The model under review builds one solid part; all positions refer to its coordinate system, in mm. A direction names the side the tool comes from. Coordinates: 2 decimals unless noted, no trailing zeros. Order: outer loops, then holes, each group sorted by start corner. A loop starts at its lowest first (then second) coordinate and runs counter-clockwise, first axis right, second up.
```python
from build123d import *

# Parameters (mm, degrees)
F0_R     = 7.5
F0_R_2   = 1.75
F1_DEPTH = 5.05


# Not quite as in the source:
# - a fillet or chamfer that OpenCascade refuses, or shapes differently, is made with other operations: its cross-section is extruded or revolved along the edge and cut away or added


with BuildPart() as f1:
    # F0 (on Top) → F1 (new body)
    with BuildSketch(Plane.XY):
        Circle(F0_R)
        Circle(F0_R_2, mode=Mode.SUBTRACT)
    extrude(amount=F1_DEPTH)

    # F2 (on Front) → F3 (revolve, cut)
    with BuildSketch(Plane.XZ):
        Polygon((3, 1.5), (3, 0), (7.75, 0), (7.75, 3.5), (5, 3.5), (5, 1.5), align=None)
        with BuildLine():
            Line((0, 5.05), (0, 1.8))
            ThreePointArc((0, 1.8), (3.25, 5.05), (0, 8.3))
            Line((0, 8.3), (0, 5.05))
        make_face()
    revolve(axis=Axis((0, 0, 2.525), (0, 0, 1)), mode=Mode.SUBTRACT)

    # F4: chamfer of 2 on 1 edges, made by hand

    # F4_s1 → F4_t2 (revolve, cut)
    with BuildSketch(Plane.XZ):
        with BuildLine():
            Line((4.8541219597, 5.05), (3.0049326417, 3.8119047619))
            ThreePointArc((3.0049326417, 3.8119047619), (3.1823683685, 4.3904307714), (3.25, 5.05))
            Line((3.25, 5.05), (4.8541219597, 5.05))
        make_face()
    revolve(axis=Axis((0, 0, 5.05), (0, 0, 1)), mode=Mode.SUBTRACT)


solid = f1.part
```
(1) For pin 1 Ø8 at (x, y) = (-1, -1.5) entering from -Z; pin 2 Ø3 at (x, y) = (-5, -0.5) entering from -Z; pin 3 Ø2 at (y, z) = (0.5, 1) entering from -X; pin 4 Ø2 at (x, y) = (0, 0) entering from +Z, all flat-tipped, find the tip position at first contact; note any pin that passes through.
A:
pin 1: stops at z = 0
pin 2: stops at z = 1.5
pin 3: stops at x = -5
pin 4: passes through
(2) Machinability: for faces 1 (the face through (0, -2, 0)), 2 (the face through (-1.08, -4.88, 2.49)), which of the approach directions +Z, -Z, +X, -X, +Y, -Y give a long, thin tool a straight path to every point of the face, cutting with its end or side? Answer none if there is none.
A:
face 1: -Z, +X, -X, +Y, -Y
face 2: -Z
(3) Wall thickness on probe 1 along Y at (x, z) = (0, 0.9); probe 2 along Z at (x, y) = (-6, 4.25); probe 3 along Z at (x, y) = (2.75, 4): over which ranges is each line inside the solid? List them lowest first.
A:
probe 1: y = -3 to -1.75, 1.75 to 3
probe 2: z = 3.5 to 5.05
probe 3: z = 1.5 to 5.05
(4) We need section A-A, the plane y = 0. Write out the cut boundary in (x, z), and give its area (3 significant figures).
A:
outline: (-7.5, 3.5) - (-5, 3.5) - (-5, 1.5) - (-3, 1.5) - (-3, 0) - (-1.75, 0) - (-1.75, 2.31) arc R3.25 cw to (-3, 3.81) - (-4.85, 5.05) - (-7.5, 5.05) - close; (1.75, 0) - (3, 0) - (3, 1.5) - (5, 1.5) - (5, 3.5) - (7.5, 3.5) - (7.5, 5.05) - (4.85, 5.05) - (3, 3.81) arc R3.25 cw to (1.75, 2.31) - close
area: 26.9 mm2
(5) We need section D-D, the plane y = -5.5. Write out the cut boundary in (x, z).
A:
outline: (-5.1, 3.5) - (5.1, 3.5) - (5.1, 5.05) - (-5.1, 5.05) - close
(6) We need section C-C, the plane z = 1.7. Write out the cut boundary in (x, y).
A:
outline: circle Ø10 at (0, 0); hole circle Ø3.5 at (0, 0)
